```python
from build123d import *

# Parameters (mm, degrees)
SKETCH_1_W          = 15
SKETCH_1_H          = 10
EXTRUDE_1_DEPTH     = 3
SKETCH_2_W          = 3
SKETCH_2_H          = 10
EXTRUDE_2_DEPTH     = 12
SKETCH_3_R          = 1.55
CUT_EXTRUDE_1_DEPTH = 18.5
SKETCH_4_R          = 1.5
CUT_EXTRUDE_2_DEPTH = 22.794494718


with BuildPart() as part:
    # 草图1 → 凸台-拉伸1 (new body)
    with BuildSketch(Plane.XY):
        Rectangle(SKETCH_1_W, SKETCH_1_H)
    extrude(amount=EXTRUDE_1_DEPTH)

    # 草图2 → 凸台-拉伸2 (add)
    with BuildSketch(Plane.XY.offset(3)):
        with Locations((-6, 0)):
            Rectangle(SKETCH_2_W, SKETCH_2_H)
    extrude(amount=EXTRUDE_2_DEPTH)

    # 草图3 → 切除-拉伸1 (cut, through all)
    with BuildSketch(Plane(origin=(0, 0, 0), x_dir=(-1, 0, 0), z_dir=(0, 0, -1))):
        with Locations((-2.5, 0)):
            Circle(SKETCH_3_R)
    extrude(amount=-CUT_EXTRUDE_1_DEPTH, mode=Mode.SUBTRACT)

    # 草图4 → 切除-拉伸2 (cut, through all)
    with BuildSketch(Plane.ZY.offset(7.5)):
        with Locations((10, 0)):
            Circle(SKETCH_4_R)
    extrude(amount=-CUT_EXTRUDE_2_DEPTH, mode=Mode.SUBTRACT)


solid = part.part
```
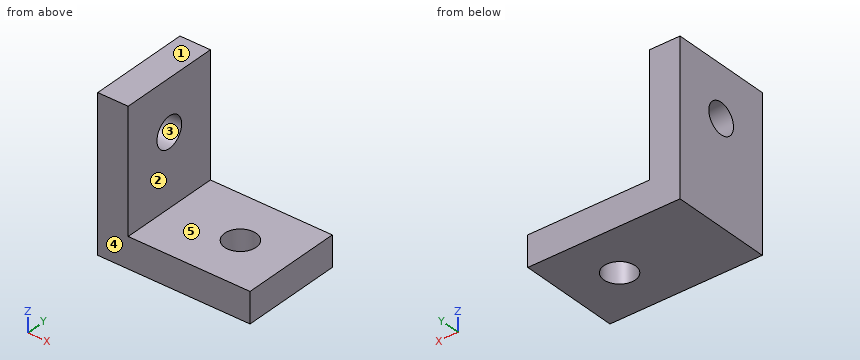
The listing builds one solid part. Answer for the finished solid, in the listing's coordinates (mm). Face numbers are marked on the shaded views. A direction names the side the tool comes from. Coordinates: 2 decimals unless noted, no trailing zeros. Loops run counter-clockwise (first coordinate to the right, second up) from the corner with the lowest first, then second, coordinate; pieces in that order, holes last. Notation, with made-up numbers: M 6,-19 L 56,-19 A22 ccw 56,16 Z; hole C 33.25,63.5 d1. An arc over 180 degrees is marked long. Answer as CSV lines item,"result". Start each with the question number.
(1) The part is cut by section D-D (z = 2.25). Give the vertices of the cut face in (x, y).
(2) The part is cut by section C-C (y = 0). Give the vertices of the cut face in (x, z).
(3) The part is cut by section B-B (z = 10). Give the vertices of the cut face in (x, y), and give its area (3 significant figures).
(4) The mould has two halves that part along Y. Classify the marked faces 3, 4 and 5: pulls with the +Y half, pulls with the -Y half, needs draft (parallel to the pull), parting line crosses it, or undercut.
(5) For the marked faces 1 and 2, determine the directions among +Z, -Z, +X, -X, +Y, -Y from which every point of the face is accessible in a straight line to the end or side of a thin tool.
(6) Find the intervals of material crossed by L1, parallel to Y at x = -5.85, z = 10; L2, parallel to X at y = 4.75, z = 9.75; L3, parallel to Z at x = -2, y = -3, in increasing order. Write a range as [from, to].
(7) The part is cut by section A-A (x = 2.5). Give the vertices of the cut face in (y, z).
(8) Given pin 1 (4 mm diameter, centred on y = -3, z = 12.5, fed in from +X); pin 2 (1.5 mm diameter, centred on x = 5.5, z = 4, fed in from -Y); pin 3 (5 mm diameter, centred on x = 5.5, y = -2, fed in from +Z), each flat-ended and moving along its own axis, determine where each tip first touches the part or whether it passes through.
Determined:
1,outline,"M -7.5,-5 L 7.5,-5 L 7.5,5 L -7.5,5 Z; hole C 2.5,0 d3.1"
2,outline,"M -7.5,0 L 0.95,0 L 0.95,3 L -4.5,3 L -4.5,8.5 L -7.5,8.5 Z; M -7.5,11.5 L -4.5,11.5 L -4.5,15 L -7.5,15 Z; M 4.05,0 L 7.5,0 L 7.5,3 L 4.05,3 Z"
3,outline,"M -7.5,-5 L -4.5,-5 L -4.5,-1.5 L -7.5,-1.5 Z; M -7.5,1.5 L -4.5,1.5 L -4.5,5 L -7.5,5 Z"
3,area,"21.0 mm2"
4,face 3,"undercut"
4,face 4,"pulls with the -Y half"
4,face 5,"needs draft"
5,face 1,"+Z, +X, -X, +Y, -Y"
5,face 2,"+Z, +X, +Y, -Y"
6,L1,"[-5, -1.5], [1.5, 5]"
6,L2,"[-7.5, -4.5]"
6,L3,"[0, 3]"
7,outline,"M -5,0 L -1.55,0 L -1.55,3 L -5,3 Z; M 1.55,0 L 5,0 L 5,3 L 1.55,3 Z"
8,pin 1,"x = -4.5"
8,pin 2,"through"
8,pin 3,"z = 3"
